```python
from build123d import *

# Parameters (mm, degrees)
SKETCH1_R               = 5
SKETCH1_R_2             = 1.65
BOSS_EXTRUDE1_DEPTH     = 3
FILLET1_R               = 2.5
SKETCH2_W               = 10
SKETCH2_H               = 3
CUT_EXTRUDE1_DEPTH      = 1
CUT_EXTRUDE1_DEPTH_BACK = 4
BOSS_EXTRUDE2_DEPTH     = 3
SKETCH4_R               = 2
SKETCH4_W               = 3.05
SKETCH4_H               = 15
CUT_EXTRUDE2_DEPTH      = 1
CUT_EXTRUDE2_DEPTH_BACK = 4


with BuildPart() as part:
    # Sketch1 → Boss-Extrude1 (new body)
    with BuildSketch(Plane(origin=(0, 0, 0), x_dir=(0, 0, -1), z_dir=(1, 0, 0))):
        with BuildLine():
            Line((-20, -147), (-20, 0))
            ThreePointArc((-20, 0), (-2.849659193, 19.795945102), (19.187944249, 5.641169694))
            Line((19.187944249, 5.641169694), (63.181778112, -144))
            Line((63.181778112, -144), (63.181778112, -147))
            Line((63.181778112, -147), (-20, -147))
        make_face()
        Circle(SKETCH1_R, mode=Mode.SUBTRACT)
        with Locations((0, -25)):
            Circle(SKETCH1_R_2, mode=Mode.SUBTRACT)
        Polygon((5, -34.733881779), (5, -122), (30.655848018, -122), align=None, mode=Mode.SUBTRACT)
        Polygon((10.262540517, -25.557391536), (3.923266591, -11.962774731), (6.642189952, -10.694919945), (12.981463878, -24.289536751), align=None, mode=Mode.SUBTRACT)
        Polygon((-12.981463878, -24.289536751), (-6.642189952, -10.694919945), (-3.923266591, -11.962774731), (-10.262540517, -25.557391536), align=None, mode=Mode.SUBTRACT)
    extrude(amount=BOSS_EXTRUDE1_DEPTH)

    # Fillet1
    fillet1_edges = [part.edges().sort_by_distance(p)[0] for p in [
        (1.5, -122, -30.655848018),
        (1.5, -34.733881779, -5),
        (1.5, -122, -5),
    ]]
    fillet(fillet1_edges, radius=FILLET1_R)

    # Sketch2 → Cut-Extrude1 (cut, two sides)
    with BuildSketch(Plane(origin=(3, 0, 0), x_dir=(0, 0, -1), z_dir=(1, 0, 0))) as cut_extrude1_sk:
        with Locations((45.681778112, -145.5)):
            Rectangle(SKETCH2_W, SKETCH2_H)
        with Locations((-5, -145.5)):
            Rectangle(SKETCH2_W, SKETCH2_H)
    extrude(amount=CUT_EXTRUDE1_DEPTH, mode=Mode.SUBTRACT)
    extrude(cut_extrude1_sk.sketch, amount=-CUT_EXTRUDE1_DEPTH_BACK, mode=Mode.SUBTRACT)

    # Sketch2<3> → Boss-Extrude2 (add)
    with BuildSketch(Plane(origin=(3, 0, 0), x_dir=(0, 0, -1), z_dir=(1, 0, 0))):
        Polygon((50.681778112, -147), (40.681778112, -147), (28.181778112, -147), (28.181778112, -150), (63.181778112, -150), (63.181778112, -147), align=None)
    extrude(amount=-BOSS_EXTRUDE2_DEPTH)

    # Sketch4 → Cut-Extrude2 (cut, two sides)
    with BuildSketch(Plane(origin=(3, 0, 0), x_dir=(0, 0, -1), z_dir=(1, 0, 0))) as cut_extrude2_sk:
        with Locations((27, -131)):
            Circle(SKETCH4_R)
        Polygon((32.450844249, -89.195152346), (28.219966978, -74.804194159), (31.146128476, -73.943915781), (35.377005747, -88.334873967), align=None)
        with Locations((-7.5, -85.800411334)):
            Rectangle(SKETCH4_W, SKETCH4_H)
    extrude(amount=CUT_EXTRUDE2_DEPTH, mode=Mode.SUBTRACT)
    extrude(cut_extrude2_sk.sketch, amount=-CUT_EXTRUDE2_DEPTH_BACK, mode=Mode.SUBTRACT)


solid = part.part
```
The model under review builds one solid part; all positions refer to its coordinate system, in mm. A direction names the side the tool comes from. Give positions to 0.01 mm unless a question says otherwise; leave off trailing zeros. Loops run counter-clockwise (first coordinate to the right, second up) from the corner with the lowest first, then second, coordinate; pieces in that order, holes last. Notation, with made-up numbers: (-10.75, -37) - (14.25, -37) arc R12 cw to (14.25, -21) - close; hole circle Ø5 at (35.5, 78.25). An arc over 180 degrees is marked (long way). Answer as a JSON object with one key per item and string values.
Q1. Insertion check: pin 1 (1.5 mm diameter, centred on x = 2, z = 8, fed in from +Y); pin 2 (0.9 mm diameter, centred on x = 2, y = -81.5, fed in from -Z); pin 3 (0.9 mm diameter, centred on x = 2, z = 6.5, fed in from -Y). Each pin has a flat end and moves straight along its axis. Give the tip position at first contact, or say it passes through.
Worked out:
{"pin 1": "stops at y = 18.64", "pin 2": "stops at z = -44.94", "pin 3": "stops at y = -144"}
Q2. For faces 1 (the flat face through (2, -147, -63.182)), 2 (the flat face through (2, -147, -46)), 3 (the flat face through (2, -144, 5)), list the 3-axis set-ups (+Z, -Z, +X, -X, +Y, -Y) from which the entire face can be reached by the end or side of a thin tool; tool diameter is ignored.
Worked out:
{"face 1": "-Z, +X, -X, +Y, -Y", "face 2": "+X, -X", "face 3": "+X, -X, -Y"}
Q3. Add section A-A on y = -112. State the section outline as (x, z) points, plus the area to 3 significant figures.
Worked out:
{"outline": "(0, -53.77) - (3, -53.77) - (3, -27.72) - (0, -27.72) - close; (0, -5) - (3, -5) - (3, 20) - (0, 20) - close", "area": "153 mm^2"}
Q4. Add section D-D on z = -55.5. State the section outline as (x, y) points.
Worked out:
{"outline": "(0, -150) - (3, -150) - (3, -117.87) - (0, -117.87) - close"}
Q5. Add section B-B on z = -47. State the section outline as (x, y) points, plus the area to 3 significant figures.
Worked out:
{"outline": "(0, -150) - (3, -150) - (3, -147) - (0, -147) - close; (0, -144) - (3, -144) - (3, -88.96) - (0, -88.96) - close", "area": "174 mm^2"}
Q6. To check wall thickness, follow line 1 along Z through (x, y) = (1.7, -21); line 2 along Z through (x, y) = (1, -75); line 3 along Z through (x, y) = (0.7, -131). State the ranges of each line that lie inside material, in increasing order.
Worked out:
{"line 1": "z = -27.02 to -11.45, -8.14 to 8.14, 11.45 to 20", "line 2": "z = -42.9 to -31.46, -28.28 to -16.84, -5 to 20", "line 3": "z = -59.36 to -29, -25 to 20"}
Q7. Add section C-C on x = 1.5. Count the separate pieces of the cut face and the enclosed holes in it, plus the area to 3 significant figures.
Worked out:
{"separate pieces": "1", "enclosed holes": "9", "area": "8,490 mm^2"}
Q8. Mouldability with a two-part tool opening along Y and no side actions: class faces 4 (the flat face through (3, -64, -3)), 5 (the flat face through (2, -150, -45)), 6 (the cylindrical face through (1.52, -49.62, -7.19)) as +Y half, -Y half, draft (parallel to the pull), parting line (faces both ways), or undercut.
Worked out:
{"face 4": "draft", "face 5": "-Y half", "face 6": "undercut"}
